Design review of the part shown in the three views and the two pictorial views. Dimensions are in mm from the part's minimum x, y and z. Round coordinates to 2 decimals unless told otherwise and drop trailing zeros. Write each loop counter-clockwise with the first axis right and the second up, starting at its lowest first coordinate (ties: lowest second). Pieces come first, ordered by that corner, then holes. Notation, with made-up numbers: (5, 5) -> (30, 5) arc R31 cw to (30, 44) -> close; hole circle Ø3 at (45.25, -3). An arc over 180 degrees is marked (long way). Answer as a JSON object with one key per item and string values. Group by question number.
1) We need section A-A, the plane z = 1.35. Write out the cut boundary in (x, y), then the cut area to 3 significant figures.
2) We need section C-C, the plane y = 57.5. Write out the cut boundary in (x, z).
3) To check wall thickness, follow probe 1 along Y at (x, z) = (62, 0.9); probe 2 along Y at (x, z) = (47, 0.75) (1 decimal); probe 3 along X at (y, z) = (32, 1.9) (1 decimal). State the ranges of each line that lie inside material, in increasing order. Write a range as [from, to].
4) We need section B-B, the plane x = 12. Write out the cut boundary in (y, z), then the cut area to 3 significant figures.
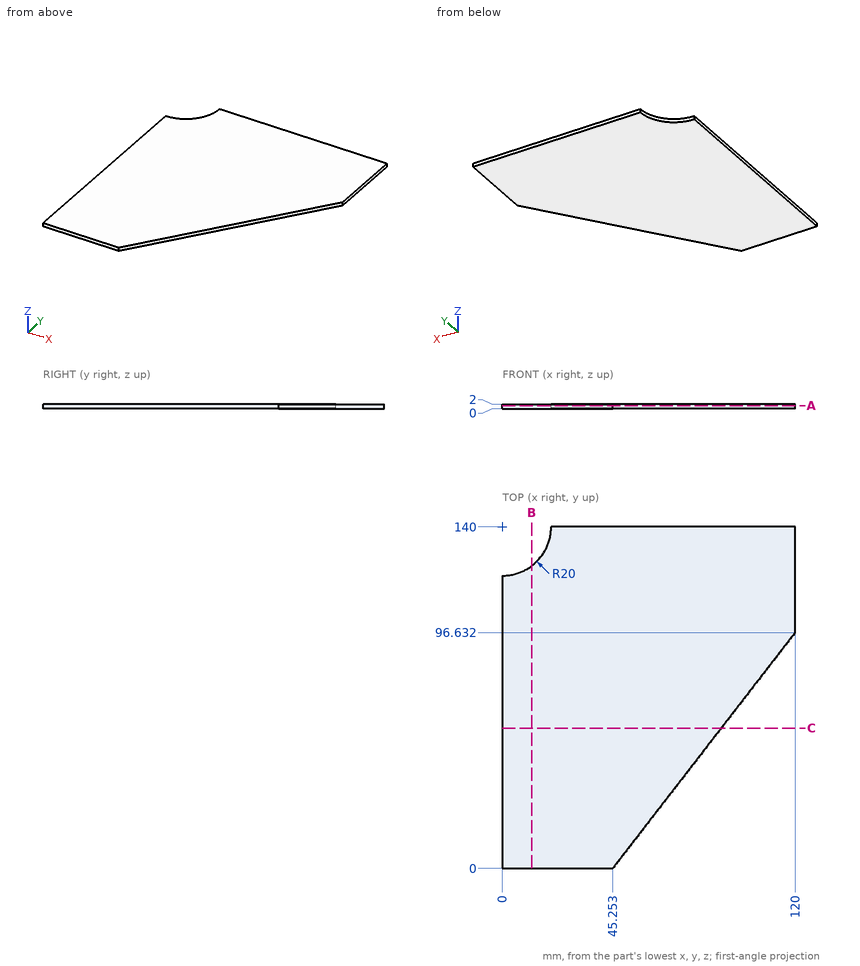
Here are the results:
{
 "1": {"outline": "(0, 0) -> (45.25, 0) -> (120, 96.63) -> (120, 140) -> (20, 140) arc R20 cw to (0, 120) -> close", "area": "12,900 mm^2"},
 "2": {"outline": "(0, 0) -> (89.73, 0) -> (89.73, 2) -> (0, 2) -> close"},
 "3": {"probe 1": "y = [21.65, 140]", "probe 2": "y = [2.3, 140]", "probe 3": "x = [0, 70]"},
 "4": {"outline": "(0, 0) -> (124, 0) -> (124, 2) -> (0, 2) -> close", "area": "248 mm^2"}
}
